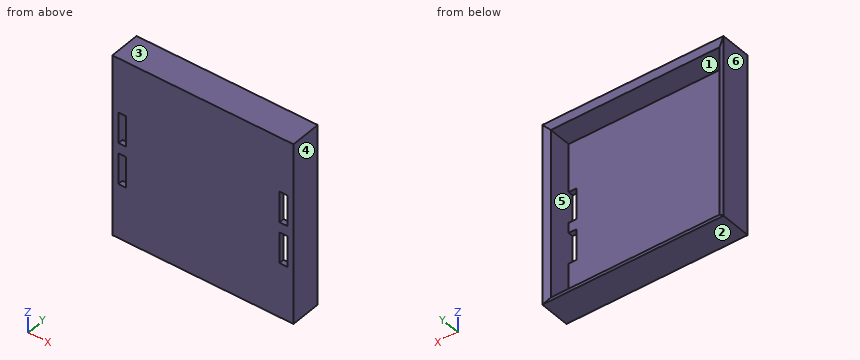
Autodesk Inventor part; units mm, degrees
ref_plane "YZ Plane" through (0, 0, 0) normal (1, 0, 0) x (0, 1, 0)
ref_plane "XZ Plane" through (0, 0, 0) normal (0, 1, 0) x (-1, 0, 0)
ref_plane "XY Plane" through (0, 0, 0) normal (0, 0, 1) x (1, 0, 0)
sketch "Sketch1" plane through (0, 0, 0) normal (0, 1, 0) x (-1, 0, 0)
  point P0 (0, 0)
sketch "Sketch2" plane through (0, 0, 0) normal (0, 1, 0) x (-1, 0, 0)
  line L0 (0, 0) -> (35.2, 0)
  line L1 (35.2, 0) -> (35.2, -35.2)
  line L2 (35.2, -35.2) -> (0, -35.2)
  line L3 (0, -35.2) -> (0, 0)
  dimension "d0" = 35.2
  dimension "d1" = 35.2
extrude "Extrusion1" add sketch "Sketch2" along normal blind 1
sketch "Sketch3" plane through (0, 1, 0) normal (0, 1, 0) x (1, 0, 0)
  line L0 (0, 35.2) -> (-35.2, 35.2)
  line L1 (-35.2, 35.2) -> (-35.2, 0)
  line L2 (-35.2, 0) -> (0, 0)
  line L3 (0, 0) -> (0, 35.2)
  line L4 (-35.2, 0) -> (0, 0)
  line L5 (0, 0) -> (-1.2, 0)
  line L6 (-1.2, 0) -> (-1.2, 1.2)
  line L7 (-1.2, 1.2) -> (-34, 1.2)
  line L8 (-34, 1.2) -> (-34, 34)
  line L9 (-34, 34) -> (-1.2, 34)
  line L10 (-1.2, 34) -> (-1.2, 1.2)
  dimension "d4" = 1.2
  dimension "d5" = 1.2
  dimension "d6" = 32.8
  dimension "d7" = 32.8
extrude "Extrusion2" add sketch "Sketch3" along normal blind 5
sketch "Sketch4" plane through (0, 1, 0) normal (0, 1, 0) x (1, 0, 0)
  line L0 (-1.2, 1.2) -> (-1.2, 34)
  line L1 (-1.2, 34) -> (-34, 34)
  line L2 (-34, 34) -> (-34, 1.2)
  line L3 (-34, 1.2) -> (-1.2, 1.2)
  line L4 (-1.2, 1.2) -> (-1.2, 34)
  line L5 (-1.2, 17.6) -> (-34, 17.6)
  line L6 (-34, 34) -> (-1.2, 34)
  line L7 (-17.6, 34) -> (-17.6, 1.2)
  line L8 (-17.6, 17.6) -> (-17.6, 18.6)
  line L9 (-34, 17.6) -> (-34, 17.6)
  line L10 (-34, 1.2) -> (-34, 34)
  line L11 (-34, 17.6) -> (-32.5, 17.6)
  line L12 (-1.2, 17.6) -> (-1.2, 18.6)
  line L13 (-1.2, 18.6) -> (-2.7, 18.6)
  line L14 (-2.7, 18.6) -> (-2.7, 24.6)
  line L15 (-2.7, 24.6) -> (-1.2, 24.6)
  line L16 (-1.2, 17.6) -> (-1.2, 15.6)
  line L17 (-1.2, 17.6) -> (-1.2, 16.6)
  line L18 (-1.2, 34) -> (-1.2, 1.2)
  line L19 (-1.2, 16.6) -> (-2.7, 16.6)
  line L20 (-2.7, 16.6) -> (-2.7, 10.6)
  line L21 (-2.7, 10.6) -> (-1.2, 10.6)
  line L22 (-34, 17.6) -> (-34, 18.6)
  line L23 (-34, 1.2) -> (-34, 34)
  line L24 (-34, 18.6) -> (-32.5, 18.6)
  line L25 (-32.5, 18.6) -> (-32.5, 24.6)
  line L26 (-32.5, 24.6) -> (-34, 24.6)
  line L27 (-34, 17.6) -> (-34, 16.6)
  line L28 (-34, 16.6) -> (-32.5, 16.6)
  line L29 (-32.5, 16.6) -> (-32.5, 10.6)
  line L30 (-32.5, 10.6) -> (-34, 10.6)
  point P0 (0, 0)
  point P1 (-34, 23.6)
  dimension "d13" = 1
  dimension "d19" = 1.5
  dimension "d20" = 6
  dimension "d49" = 6
extrude "Extrusion3" cut sketch "Sketch4" against normal blind 4 contours L21 L20 L19 L0 | L2 L28 L29 L30 | L13 L14 L15 L0 | L2 L26 L25 L24
chamfer "Chamfer3" distance 1.2 distance2 0.6 1 edges at (-1.2, 6, -17.6) measured on face at (-34.8, 6, -23.0667)
chamfer "Chamfer4" distance 1.2 distance2 0.6 1 edges at (-17.6, 6, -1.2) measured on face at (-34.8, 6, -23.0667)
chamfer "Chamfer5" distance 1.2 distance2 0.6 1 edges at (-17.6, 6, -34) measured on face at (-34.8, 6, -23.0667)
chamfer "Chamfer6" distance 1.2 distance2 0.6 1 edges at (-34, 6, -17.6) measured on face at (-34.8, 6, -23.0667)
properties part number "led-compartment-2"
Read the model definition and answer for the solid it produces. Units are mm, in the model's axes. Face numbers are marked on the shaded views. A direction names the side the tool comes from. Coordinates: 2 decimals unless noted, no trailing zeros. Write each loop counter-clockwise with the first axis right and the second up, starting at its lowest first coordinate (ties: lowest second). Pieces come first, ordered by that corner, then holes. Notation, with made-up numbers: (27, -12) -> (46, -12) arc R22 cw to (46, 18) -> close; hole circle Ø10 at (-4.5, 76.25). An arc over 180 degrees is marked (long way). Return JSON: item names as keys, results as strings.
1. A cutting plane is placed at A-A (z = -12.5). Give the number of separate pieces and of enclosed holes in the cut face, and give its area (3 significant figures).
Found:
{"separate pieces": "3", "enclosed holes": "0", "area": "43.5 mm2"}
2. Determine the mould class of the marked faces 1, 2, 3 and 4 for opening direction Z: pulls with the +Z half, pulls with the -Z half, needs draft (parallel to the pull), parting line crosses it, or undercut.
Found:
{"face 1": "undercut", "face 2": "pulls with the -Z half", "face 3": "pulls with the +Z half", "face 4": "needs draft"}
3. A cutting plane is placed at B-B (y = 4.25). Determine the outline of the cut face in (x, z).
Found:
{"outline": "(-35.2, -35.2) -> (0, -35.2) -> (0, 0) -> (-35.2, 0) -> close; hole (-34, -34) -> (-1.2, -34) -> (-1.2, -1.2) -> (-34, -1.2) -> close"}
4. A tool of negligible diameter and unlimited length cuts with its end or side. For the marked faces 5 and 6, from which of +Z, -Z, +X, -X, +Y, -Y can it reach the whole face along a straight path? Write none if from no direction.
Found:
{"face 5": "+Y", "face 6": "+Z, -Z, -X, +Y, -Y"}
5. Find the intervals of material crossed by line 1 along X through (y, z) = (3.25, -19.5); line 2 along X through (y, z) = (0.5, -20.5), in increasing order. Write a range as from..to.
Found:
{"line 1": "-35.2..-34, -1.2..0", "line 2": "-35.2..-34, -32.5..-2.7, -1.2..0"}
